from build123d import *

# Parameters (mm, degrees)
F1_DEPTH = 45
F2_R     = 1.5
F3_DEPTH = 6
F4_R     = 1.5
F5_DEPTH = 6


with BuildPart() as f1:
    # F0 (on Top) → F1 (new body)
    with BuildSketch(Plane.XY):
        Polygon((3, -1.7320508076), (3, 1.7320508076), (0, 3.4641016151), (-3, 1.7320508076), (-3, -1.7320508076), (0, -3.4641016151), align=None)
    extrude(amount=F1_DEPTH)

    # F2 (on face) → F3 (join)
    with BuildSketch(Plane.XY.offset(45)):
        Circle(F2_R)
    extrude(amount=F3_DEPTH)

    # F4 (on face) → F5 (cut)
    with BuildSketch(Plane(origin=(0, 0, 0), x_dir=(1, 0, 0), z_dir=(0, 0, -1))):
        Circle(F4_R)
    extrude(amount=-F5_DEPTH, mode=Mode.SUBTRACT)


solid = f1.part
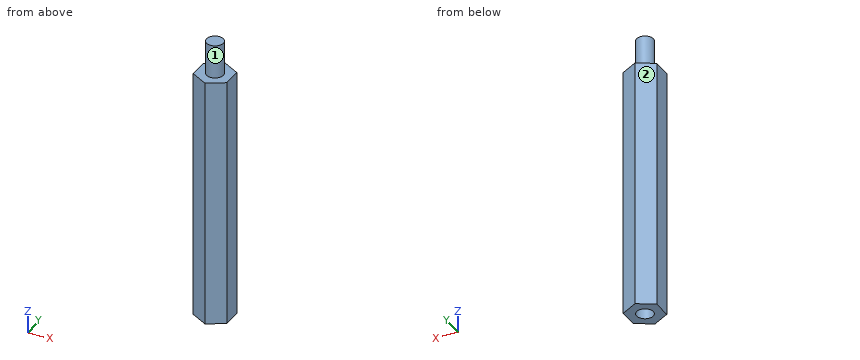
The listing builds one solid part. Answer for the finished solid, in the listing's coordinates (mm). Face numbers are marked on the shaded views. A direction names the side the tool comes from. Coordinates: 2 decimals unless noted, no trailing zeros. Loops run counter-clockwise (first coordinate to the right, second up) from the corner with the lowest first, then second, coordinate; pieces in that order, holes last. Notation, with made-up numbers: M 27.5,82 L 36.5,82 A10 cw 36.5,94 Z; hole C 50.25,-27 d1. An arc over 180 degrees is marked long. Answer in a Markdown table with one row per item.
1) Find section C-C (x = 2.25). Determine the outline of the cut face in (y, z).
Answers below:
| item | result |
|---|---|
| outline | M -2.17,0 L 2.17,0 L 2.17,45 L -2.17,45 Z |
2) Find the intervals of material crossed by probe 1 along Y at (x, z) = (0, 4.6); probe 2 along X at (y, z) = (0, 4.7); probe 3 along Z at (x, y) = (-1.75, -0.75), in increasing order.
Answers below:
| item | result |
|---|---|
| probe 1 | -3.46 to -1.5, 1.5 to 3.46 |
| probe 2 | -3 to -1.5, 1.5 to 3 |
| probe 3 | 0 to 45 |
3) Which of the six approach directions +Z, -Z, +X, -X, +Y, -Y give full straight-line access (tool end or side, diameter ignored) to the marked faces 1 and 2?
Answers below:
| item | result |
|---|---|
| face 1 | +Z |
| face 2 | +Z, -Z, -X, +Y |
4) Find section A-A (y = 0). Determine the outline of the cut face in (x, z), then the cut area to 3 significant figures.
Answers below:
| item | result |
|---|---|
| outline | M -3,0 L -1.5,0 L -1.5,6 L 1.5,6 L 1.5,0 L 3,0 L 3,45 L 1.5,45 L 1.5,51 L -1.5,51 L -1.5,45 L -3,45 Z |
| area | 270 mm^2 |
5) Find section D-D (y = 2.25). Determine the outline of the cut face in (x, z), then the cut area to 3 significant figures.
Answers below:
| item | result |
|---|---|
| outline | M -2.1,0 L 2.1,0 L 2.1,45 L -2.1,45 Z |
| area | 189 mm^2 |
6) Find section B-B (z = 20). Determine the outline of the cut face in (x, y).
Answers below:
| item | result |
|---|---|
| outline | M -3,-1.73 L 0,-3.46 L 3,-1.73 L 3,1.73 L 0,3.46 L -3,1.73 Z |
